Geometry: see drawing. Coordinates: mm, zero at the bounding-box minimum. A direction names the side the tool comes from. Give positions to 0.01 mm unless a question says otherwise; leave off trailing zeros. Write each loop counter-clockwise with the first axis right and the second up, starting at its lowest first coordinate (ties: lowest second). Pieces come first, ordered by that corner, then holes. Notation, with made-up numbers: M 16.25,46.5 L 22.25,46.5 A7 cw 22.25,50.5 Z; hole C 1.25,16 d2. An arc over 180 degrees is marked long. Use a Markdown table: item, result. Add a question column.
(1) Cut plane C-C (z = 4). Output: boundary loops of the cut face in (x, y).
(2) Pin query (flat end, axial travel): pin 1 Ø17 at (y, z) = (28.5, 51.5) entering from +X; pin 2 Ø12 at (y, z) = (46, 51.5) entering from -X; pin 3 Ø20 at (x, y) = (14.5, 28.5) entering from +Z. Return the tip coordinate at first contact, or that it passes through.
(3) Cut plane A-A (z = 33.5). Output: boundary loops of the cut face in (x, y).
(4) Cut plane D-D (x = 41). Output: boundary loops of the cut face in (y, z), plus the area to 3 significant figures.
(5) Material intervals for L1, parallel to X at y = 26, z = 54; L2, parallel to X at y = 31.5, z = 6; L3, parallel to Z at x = 66, y = 27.5, sorted ascending.
(6) Reachability of the marked faces 5, 6, 7, 8 and 9 from +Z, -Z, +X, -X, +Y, -Y: full face, straight path, thin tool, end or side. Return the list, or none.
(7) Draft query along X for the marked faces 1, 2, 3 and 4. Return one class per face: released by +X, released by -X, zero draft, split by the parting line, or undercut.
(8) Cut plane B-B (y = 3). Output: boundary loops of the cut face in (x, z).
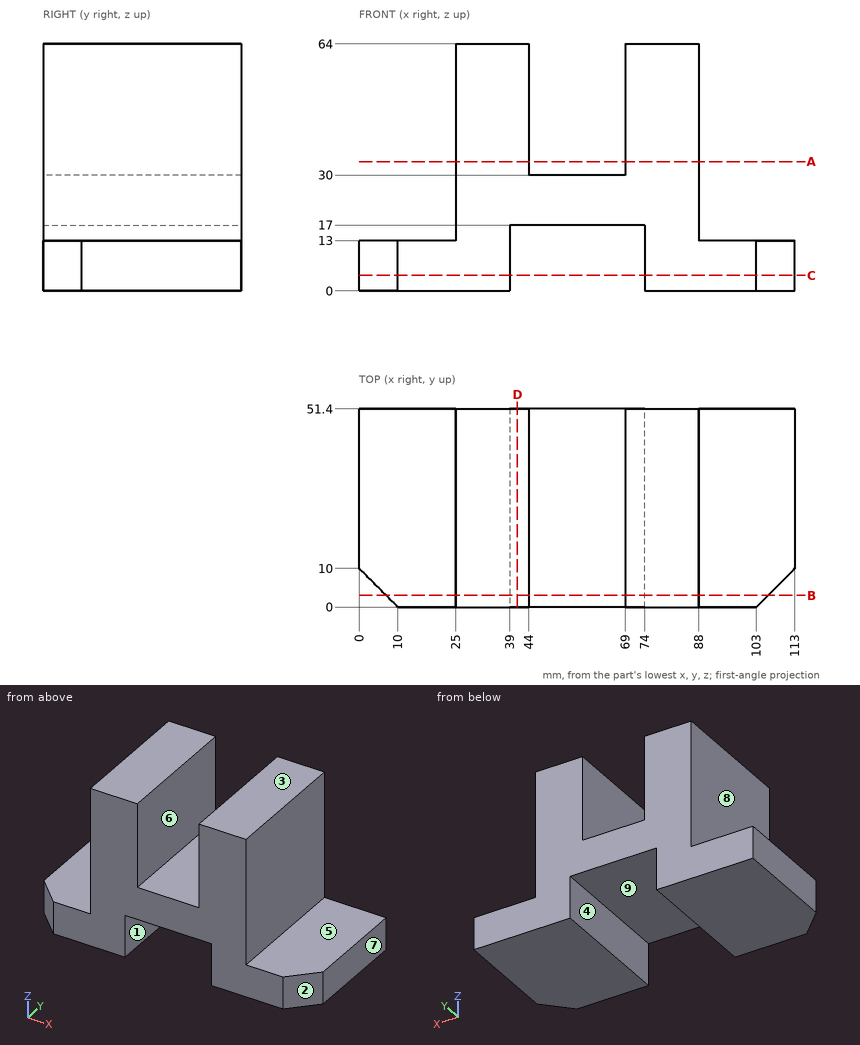
Answer list:
| question | item | result |
|---|---|---|
| 1 | outline | M 0,10 L 10,0 L 39,0 L 39,51.4 L 0,51.4 Z; M 74,0 L 103,0 L 113,10 L 113,51.4 L 74,51.4 Z |
| 2 | pin 1 | x = 88 |
| 2 | pin 2 | x = 25 |
| 2 | pin 3 | z = 13 |
| 3 | outline | M 25,0 L 44,0 L 44,51.4 L 25,51.4 Z; M 69,0 L 88,0 L 88,51.4 L 69,51.4 Z |
| 4 | outline | M 0,17 L 51.4,17 L 51.4,64 L 0,64 Z |
| 4 | area | 2,420 mm² |
| 5 | L1 | 25 to 44, 69 to 88 |
| 5 | L2 | 0 to 39, 74 to 113 |
| 5 | L3 | 17 to 30 |
| 6 | face 5 | +Z, +X, +Y, -Y |
| 6 | face 6 | +Z, +Y, -Y |
| 6 | face 7 | +Z, -Z, +X, +Y, -Y |
| 6 | face 8 | +Z, -X, +Y, -Y |
| 6 | face 9 | -Z, +Y, -Y |
| 7 | face 1 | undercut |
| 7 | face 2 | released by +X |
| 7 | face 3 | zero draft |
| 7 | face 4 | undercut |
| 8 | outline | M 7,0 L 39,0 L 39,17 L 74,17 L 74,0 L 106,0 L 106,13 L 88,13 L 88,64 L 69,64 L 69,30 L 44,30 L 44,64 L 25,64 L 25,13 L 7,13 Z |
